The model under review builds one solid part; all positions refer to its coordinate system, in mm. Give positions to 0.01 mm unless a question says otherwise; leave off trailing zeros. Loops run counter-clockwise (first coordinate to the right, second up) from the corner with the lowest first, then second, coordinate; pieces in that order, holes last. Notation, with made-up numbers: M 4.25,-26.75 L 26.25,-26.75 A24 ccw 26.25,2.25 Z; hole C 77.5,13.5 d11. An arc over 180 degrees is marked long. Write item = value, one per line. Start each with the question number.
1. We need section A-A on y = 42. Give the boundary of the cut face in (x, z).
2. We need section B-B on x = 31.75. Give the boundary of the cut face in (y, z).
3. Wall thickness on line 1 along Y through (x, z) = (31.75, 6.5); line 2 along Y through (x, z) = (29.5, 5.5); line 3 along X through (y, z) = (31, 2): over which ranges is each line inside the solid? List them lowest first. Write a range as from..to.
4. We need section C-C on z = 9.5. Give the boundary of the cut face in (x, y), then the cut area to 3 significant figures.
5. For pin 1 (1.5 mm diameter, centred on x = 48, y = 12.5, fed in from -Z); pin 2 (2 mm diameter, centred on x = 7, z = 5.5, fed in from +Y), all flat-tipped, find the tip position at first contact; note any pin that passes through.
6. Draft analysis for pull direction X (two halves, no side actions). For faces 1 (the face through (31, 26, 12.7)), 2 (the face through (58.39, 61.15, 6.44)), 3 (the face through (43.864, 45.815, 6.261)), 4 (the face through (4.85, 60.89, 6.44)), state which applies: pulls with the +X half, pulls with the -X half, needs draft (parallel to the pull), parting line crosses it, or undercut.
7. We need section D-D on x = 56. Give the boundary of the cut face in (y, z), then the cut area to 3 significant figures.
from build123d import *

# Parameters (mm, degrees)
CROQUIS1_W              = 63.5
CROQUIS1_H              = 66
CROQUIS1_R              = 12.7
SALIENTE_EXTRUIR1_DEPTH = 12.7
REDONDEO1_R             = 17


with BuildPart() as part:
    # Croquis1 → Saliente-Extruir1 (new body)
    with BuildSketch(Plane.XY):
        with Locations((31.75, 33)):
            Rectangle(CROQUIS1_W, CROQUIS1_H)
        with Locations((31.75, 42)):
            Circle(CROQUIS1_R, mode=Mode.SUBTRACT)
    extrude(amount=SALIENTE_EXTRUIR1_DEPTH)

    # Redondeo1
    redondeo1_edges = [part.edges().sort_by_distance(p)[0] for p in [
        (0, 66, 6.35),
        (63.5, 66, 6.35),
    ]]
    fillet(redondeo1_edges, radius=REDONDEO1_R)


solid = part.part
Final values:
q1.outline = M 0,0 L 19.05,0 L 19.05,12.7 L 0,12.7 Z; M 44.45,0 L 63.5,0 L 63.5,12.7 L 44.45,12.7 Z
q2.outline = M 0,0 L 29.3,0 L 29.3,12.7 L 0,12.7 Z; M 54.7,0 L 66,0 L 66,12.7 L 54.7,12.7 Z
q3.line_1 = 0..29.3, 54.7..66
q3.line_2 = 0..29.5, 54.5..66
q3.line_3 = 0..25.4, 38.1..63.5
q4.outline = M 0,0 L 63.5,0 L 63.5,49 A17 ccw 46.5,66 L 17,66 A17 ccw 0,49 Z; hole C 31.75,42 d25.4
q4.area = 3,560 mm²
q5.pin_1 = 0
q5.pin_2 = 63.42
q6.face_1 = needs draft
q6.face_2 = pulls with the +X half
q6.face_3 = undercut
q6.face_4 = pulls with the -X half
q7.outline = M 0,0 L 63.1,0 L 63.1,12.7 L 0,12.7 Z
q7.area = 801 mm²
